```python
from build123d import *

# Parameters (mm, degrees)
EXTRUDE_1_DEPTH          = 150
SKETCH_2_R               = 15.5
CUT_EXTRUDE_7_DEPTH      = 445.437847173
CUT_EXTRUDE_8_DEPTH      = 299.705540625
CUT_EXTRUDE_8_DEPTH_BACK = 299.705540625


with BuildPart() as part:
    # 草图1 → 拉伸1 (new, symmetric)
    with BuildSketch(Plane.XY):
        Polygon((-174, -6), (174, -6), (174, -175), (190, -175), (190, 175), (174, 175), (174, 6), (-174, 6), (-174, 175), (-190, 175), (-190, -175), (-174, -175), align=None)
    extrude(amount=EXTRUDE_1_DEPTH, both=True)

    # 草图2 → 拉伸7 (cut, through all)
    with BuildSketch(Plane(origin=(190, 0, 0), x_dir=(0, 0, -1), z_dir=(1, 0, 0))):
        with Locations((-100, 95)):
            Circle(SKETCH_2_R)
        with Locations((0, 95)):
            Circle(SKETCH_2_R)
        with Locations((100, 95)):
            Circle(SKETCH_2_R)
        with Locations(Location((100, -95, 0), (0, 0, 270))):
            Circle(SKETCH_2_R)
        with Locations(Location((0, -95, 0), (0, 0, 270))):
            Circle(SKETCH_2_R)
        with Locations(Location((-100, -95, 0), (0, 0, 270))):
            Circle(SKETCH_2_R)
    extrude(amount=-CUT_EXTRUDE_7_DEPTH, mode=Mode.SUBTRACT)

    # 草图3 → 拉伸8 (cut, two sides: drawn at the far end of the back side and taken through both)
    with BuildSketch(Plane(origin=(0, 0, 0), x_dir=(0, 0, -1), z_dir=(1, 0, 0)).offset(-CUT_EXTRUDE_8_DEPTH_BACK)):
        Polygon((-150, 175), (-90, 175), (-150, 145), align=None)
        Polygon((150, 145), (150, 175), (90, 175), align=None)
        Polygon((150, -175), (90, -175), (150, -145), align=None)
        Polygon((-150, -145), (-150, -175), (-90, -175), align=None)
    extrude(amount=CUT_EXTRUDE_8_DEPTH + CUT_EXTRUDE_8_DEPTH_BACK, mode=Mode.SUBTRACT)


solid = part.part
```
Geometry check sheet. Reference: the model listing, model coordinates, mm. A direction names the side the tool comes from. Coordinates: 2 decimals unless noted, no trailing zeros. Write each loop counter-clockwise with the first axis right and the second up, starting at its lowest first coordinate (ties: lowest second). Pieces come first, ordered by that corner, then holes. Notation, with made-up numbers: M 75,-33.5 L 83,-33.5 A26 cw 83,-11.5 Z; hole C 43,74 d9. An arc over 180 degrees is marked long. Use one line per item in the form item = value. Start each with the question number.
1) Section check B-B on z = -100. Enter the section's corners in (x, y), and give its area (3 significant figures).
2) Go/stop test with flat-tipped pins: pin 1 Ø1.5 at (x, z) = (90.5, 18.5) entering from +Y; pin 2 Ø5 at (x, z) = (22.5, 72.5) entering from -Y; pin 3 Ø18.5 at (y, z) = (-95, -100) entering from +X. Record where each tip stops, or that it passes through.
3) Set-up check for faces 1 (the cylindrical face through (-181.9, 105.5, 111.4)), 2 (the flat face through (174, -71, 2)), 3 (the flat face through (2, 6, 2)): record each of +Z, -Z, +X, -X, +Y, -Y from which the full face is reachable in a straight line by a thin tool's end or side.
4) Section check A-A on y = -95. State how many separate pieces and enclosed holes the cut face has, and give its area (3 significant figures).
5) Thickness scan on probe 1 along Z at (x, y) = (-181, -95); probe 2 along X at (y, z) = (16, 21); probe 3 along Y at (x, z) = (179.25, -100). Record the ranges inside material, lowest first. Write a range as from..to.
6) Section check D-D on z = 128. Enter the section's corners in (x, y).
7) Section check C-C on y = 13. Enter the section's corners in (x, z).
8) Release check for a two-part mould opening along Z. For faces 4 (the flat face through (-182, 175, 1)), 5 (the flat face through (-182, -160, 120)), 6 (the cylindrical face through (-181.888, 110.368, 2.018)), 7 (the flat face through (-1, 1, -150)) record: pulls with the +Z half, pulls with the -Z half, needs draft (parallel to the pull), parting line crosses it, or undercut.
Responses:
q1.outline = M -190,-170 L -174,-170 L -174,-110.5 L -190,-110.5 Z; M -190,-79.5 L -174,-79.5 L -174,-6 L 174,-6 L 174,-79.5 L 190,-79.5 L 190,79.5 L 174,79.5 L 174,6 L -174,6 L -174,79.5 L -190,79.5 Z; M -190,110.5 L -174,110.5 L -174,170 L -190,170 Z; M 174,-170 L 190,-170 L 190,-110.5 L 174,-110.5 Z; M 174,110.5 L 190,110.5 L 190,170 L 174,170 Z
q1.area = 13,100 mm2
q2.pin_1 = 6
q2.pin_2 = -6
q2.pin_3 = through
q3.face_1 = +X, -X
q3.face_2 = +Z, -Z, -Y
q3.face_3 = +Z, -Z, +Y
q4.separate_pieces = 8
q4.enclosed_holes = 0
q4.area = 6,620 mm2
q5.probe_1 = -150..-115.5, -84.5..-15.5, 15.5..84.5, 115.5..150
q5.probe_2 = -190..-174, 174..190
q5.probe_3 = -170..-110.5, -79.5..79.5, 110.5..170
q6.outline = M -190,-156 L -174,-156 L -174,-6 L 174,-6 L 174,-156 L 190,-156 L 190,156 L 174,156 L 174,6 L -174,6 L -174,156 L -190,156 Z
q7.outline = M -190,-150 L -174,-150 L -174,150 L -190,150 Z; M 174,-150 L 190,-150 L 190,150 L 174,150 Z
q8.face_4 = needs draft
q8.face_5 = pulls with the +Z half
q8.face_6 = undercut
q8.face_7 = pulls with the -Z half
